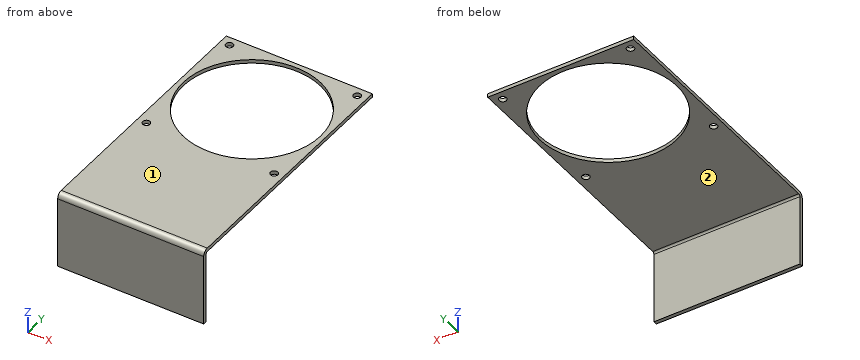
from build123d import *

# Parameters (mm, degrees)
SUPERFICIE_EXTRUIR1_1_DEPTH = 80
DAR_ESPESOR1_T1             = 2
CROQUIS2_R                  = 37.5
CROQUIS2_R_2                = 2
EXTRUIR1_DEPTH              = 80


with BuildPart() as body_1:
    # Superficie-Extruir1: a surface, the sketch's curves swept straight by 80 mm
    with BuildLine(Plane(origin=(0, 0, 0), x_dir=(0, 0, -1), z_dir=(1, 0, 0)), mode=Mode.PRIVATE) as superficie_extruir1_1_path:
        Line((0, 0), (-39, 0))
        ThreePointArc((-39, 0), (-39.707106781, 0.292893219), (-40, 1))
        Line((-40, 1), (-40, 140))
    superficie_extruir1_1 = Shell.extrude(superficie_extruir1_1_path.wire(), (1 * SUPERFICIE_EXTRUIR1_1_DEPTH, 0 * SUPERFICIE_EXTRUIR1_1_DEPTH, 0 * SUPERFICIE_EXTRUIR1_1_DEPTH))
    add(Solid.thicken(superficie_extruir1_1, DAR_ESPESOR1_T1))

    # Croquis2 → Extruir1 (cut)
    with BuildSketch(Plane.XY.offset(42)):
        with Locations((40, 100)):
            Circle(CROQUIS2_R)
        with Locations((5, 135)):
            Circle(CROQUIS2_R_2)
        with Locations(Location((75, 135, 0), (0, 0, 180))):
            Circle(CROQUIS2_R_2)
        with Locations((75, 65)):
            Circle(CROQUIS2_R_2)
        with Locations(Location((5, 65, 0), (0, 0, 180))):
            Circle(CROQUIS2_R_2)
    extrude(amount=-EXTRUIR1_DEPTH, mode=Mode.SUBTRACT)


solid = body_1.part
The model under review builds one solid part; all positions refer to its coordinate system, in mm. Face numbers are marked on the shaded views. A direction names the side the tool comes from. Give positions to 0.01 mm unless a question says otherwise; leave off trailing zeros. Write each loop counter-clockwise with the first axis right and the second up, starting at its lowest first coordinate (ties: lowest second). Pieces come first, ordered by that corner, then holes.
1. Tool access review of the marked faces 1 and 2: name each direction out of +Z, -Z, +X, -X, +Y, -Y from which nothing blocks a thin tool from reaching the whole face with its end or side.
2. Add section C-C, the plane x = 5.5. Write out the cut boundary in (y, z), plus the area to 3 significant figures.
3. Add section D-D, the plane y = 86. Write out the cut boundary in (x, z), plus the area to 3 significant figures.
4. Add section B-B, the plane x = 28. Write out the cut boundary in (y, z).
5. For P1, Ø6, axis at x = 58.5, z = 28, coming from the +Y side; P2, Ø4.5, axis at x = 75, y = 65, coming from the -Z side, all flat-tipped, find the tip position at first contact; note any pin that passes through.
6. Add section A-A, the plane y = 70. Write out the cut boundary in (x, z).
7. Wall thickness on L1, parallel to Z at x = 53, y = 4; L2, parallel to Y at x = 7, z = 34; L3, parallel to Y at x = 40, z = 40.95: over which ranges is each line inside the solid? List them lowest first.
Worked answers:
1. face 1: +Z, +X, -X, +Y, -Y
1. face 2: -Z, +X, -X, +Y
2. outline: (-2, 0) - (0, 0) - (0, 39) arc R1 cw to (1, 40) - (63.06, 40) - (63.06, 42) - (1, 42) arc R3 ccw to (-2, 39) - close; (66.94, 40) - (85.3, 40) - (85.3, 42) - (66.94, 42) - close; (114.7, 40) - (133.06, 40) - (133.06, 42) - (114.7, 42) - close; (136.94, 40) - (140, 40) - (140, 42) - (136.94, 42) - close
2. area: 288 mm2
3. outline: (0, 40) - (5.21, 40) - (5.21, 42) - (0, 42) - close; (74.79, 40) - (80, 40) - (80, 42) - (74.79, 42) - close
3. area: 20.8 mm2
4. outline: (-2, 0) - (0, 0) - (0, 39) arc R1 cw to (1, 40) - (64.47, 40) - (64.47, 42) - (1, 42) arc R3 ccw to (-2, 39) - close; (135.53, 40) - (140, 40) - (140, 42) - (135.53, 42) - close
5. P1: stops at y = 0
5. P2: stops at z = 40
6. outline: (0, 40) - (17.5, 40) - (17.5, 42) - (0, 42) - close; (62.5, 40) - (80, 40) - (80, 42) - (62.5, 42) - close
7. L1: z = 40 to 42
7. L2: y = -2 to 0
7. L3: y = -1.28 to 62.5, 137.5 to 140
